Part model, mm, in its own coordinate system. Face numbers are marked on the shaded views. A direction names the side the tool comes from. Give positions to 0.01 mm unless a question says otherwise; leave off trailing zeros. Write each loop counter-clockwise with the first axis right and the second up, starting at its lowest first coordinate (ties: lowest second). Pieces come first, ordered by that corner, then holes.
Autodesk Inventor part; units mm, degrees
ref_plane "YZ Plane" through (0, 0, 0) normal (1, 0, 0) x (0, 1, 0)
ref_plane "XZ Plane" through (0, 0, 0) normal (0, 1, 0) x (-1, 0, 0)
ref_plane "XY Plane" through (0, 0, 0) normal (0, 0, 1) x (1, 0, 0)
ref_plane "Work Plane1" through (0, 0, 0) normal (0, 0, 1) x (1, 0, 0)
sketch "Sketch2" plane through (0, 0, 0) normal (0, 0, 1) x (1, 0, 0)
  line L0 (-900, -1000) -> (900, -1000)
  line L1 (900, -1000) -> (900, 1000)
  line L2 (900, 1000) -> (-900, 1000)
  line L3 (-900, 1000) -> (-900, -1000)
  line L4 (900, -1000) -> (-900, -1000)
  line L5 (-900, -1000) -> (-900, -500)
  line L6 (-900, -1000) -> (-900, 1000)
  line L7 (-300, -500) -> (-300, -250)
  line L8 (-300, -250) -> (300, -250)
  line L9 (300, -250) -> (300, 1000)
  line L10 (-900, 1000) -> (-900, -500)
  line L11 (-300, -500) -> (-900, -500)
  point P0 (0, 0)
  point P1 (-300, -1000)
  point P2 (300, -1000)
  dimension "d4" = 600
  dimension "d5" = 600
  dimension "d6" = 600
  dimension "d7" = 500
  dimension "d8" = 1200
  dimension "d9" = 750
  dimension "d10" = 1500
extrude "Extrusion2" [suppressed]
ref_plane "Work Plane2" through (0, 0, 0) normal (0, 0, 1) x (1, 0, 0)
sketch "Sketch4" plane through (0, 0, 0) normal (0, 0, 1) x (1, 0, 0)
  line L0 (-300, -500) -> (-900, -500)
  line L1 (-900, -500) -> (-900, -1000)
  line L2 (-900, -1000) -> (900, -1000)
  line L3 (900, -1000) -> (900, 1000)
  line L4 (900, 1000) -> (300, 1000)
  line L5 (300, 1000) -> (300, -250)
  line L6 (300, -250) -> (-300, -250)
  line L7 (-300, -250) -> (-300, -500)
  line L8 (300, 1000) -> (300, -250)
  line L9 (300, -250) -> (-300, -250)
  line L10 (-300, -500) -> (-900, -500)
  line L11 (-300, -500) -> (-300, -250)
  line L12 (-900, 1000) -> (300, 1000)
  line L13 (-900, 1000) -> (-900, -500)
  point P0 (0, 0)
extrude "Extrusion4" add sketch "Sketch4" against normal blind 540 contours L0 L13 L12 L5 L6 L7
properties part number "data" material "ABS Plastic"
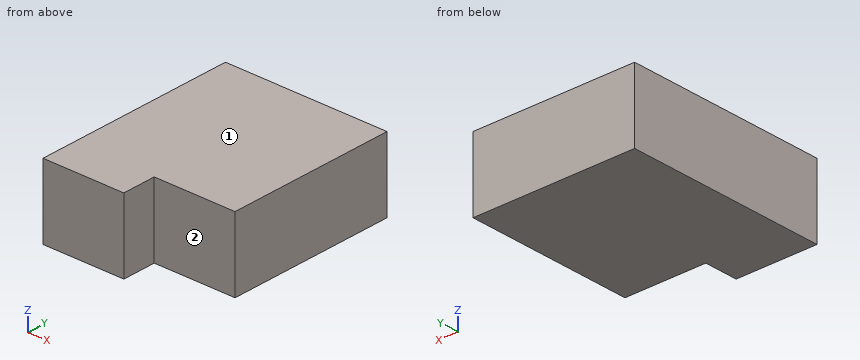
1) Saw through at B-B (z = -204.5). Write the cut outline in (x, y).
Check result:
outline: (-900, -500) - (-300, -500) - (-300, -250) - (300, -250) - (300, 1000) - (-900, 1000) - close
2) Saw through at A-A (x = -279). Write the cut outline in (y, z), and give its area (3 significant figures).
Check result:
outline: (-250, -540) - (1000, -540) - (1000, 0) - (-250, 0) - close
area: 675,000 mm2
3) 3-axis set-ups, long thin cutter, end or side, ignore diameter. For the marked faces 1 and 2: which of +Z, -Z, +X, -X, +Y, -Y reach the whole face in a straight line?
Check result:
face 1: +Z, +X, -X, +Y, -Y
face 2: +Z, -Z, +X, -Y
4) Saw through at C-C (y = -303.5). Write the cut outline in (x, z).
Check result:
outline: (-900, -540) - (-300, -540) - (-300, 0) - (-900, 0) - close
5) Drill centre lines: L1, parallel to Y at x = -287.5, z = -42; L2, parallel to X at y = -352.5, z = -461.5. Where is each one in solid material? Low to high.
Check result:
L1: y = -250 to 1000
L2: x = -900 to -300
